The figure shows three views and two pictorial views of one solid part (mm, origin at its lowest corner). Answer the questions. Coordinates: 2 decimals unless noted, no trailing zeros. Write each loop counter-clockwise with the first axis right and the second up, starting at its lowest first coordinate (ties: lowest second). Pieces come first, ordered by that corner, then holes.
Item 1: Determine the mould class of the marked faces 1 and 2 for opening direction Z: released by +Z, released by -Z, zero draft, split by the parting line, or undercut.
Item 2: Section C-C (y = 1.65) is taken. Give the vertices of the cut face in (x, z), then the cut area to 3 significant figures.
Item 3: Section B-B (x = 20) is taken. Give the vertices of the cut face in (y, z), then the cut area to 3 significant figures.
Item 4: Straight lines are drawn through the part: probe 1 along X at (y, z) = (1.35, 5); probe 2 along X at (y, z) = (1.55, 19.5); probe 3 along X at (y, z) = (0.7, 35). For each, find the intervals that lie inside material, in ascending order.
Item 5: Section A-A (z = 20) is taken. Give the vertices of the cut face in (x, y), then the cut area to 3 significant figures.
Item 6: Each of these flat-tipped pins is pushed along its axis until it touches: P1, Ø2, axis at x = 35, z = 35, coming from the -Y side; P2, Ø1, axis at x = 31, z = 8.5, coming from the +Y side. Where does it stop, or does it pass through?
Item 7: Section D-D (x = 35) is taken. Give the vertices of the cut face in (y, z), then the cut area to 3 significant figures.
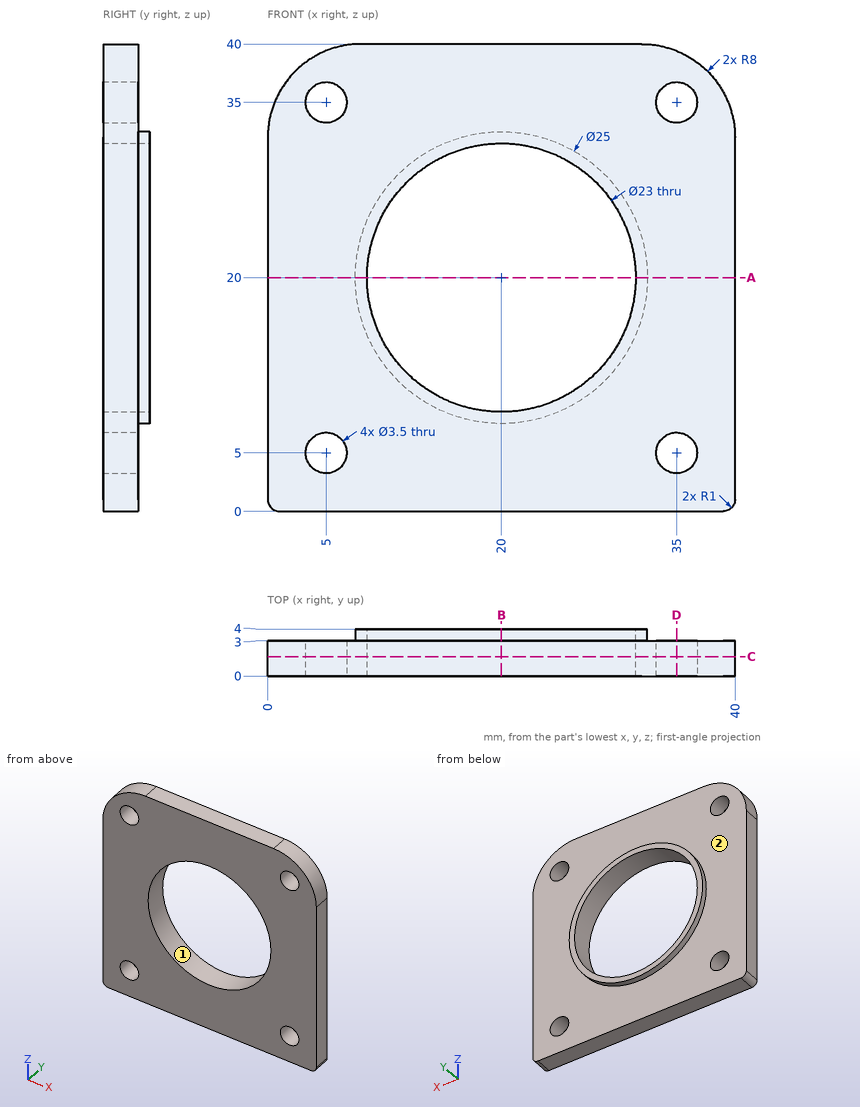
Established:
1. face 1: undercut
1. face 2: zero draft
2. outline: (0, 1) arc R1 ccw to (1, 0) - (39, 0) arc R1 ccw to (40, 1) - (40, 32) arc R8 ccw to (32, 40) - (8, 40) arc R8 ccw to (0, 32) - close; hole circle Ø3.5 at (5, 5); hole circle Ø3.5 at (5, 35); hole circle Ø23 at (20, 20); hole circle Ø3.5 at (35, 5); hole circle Ø3.5 at (35, 35)
2. area: 1,120 mm2
3. outline: (0, 0) - (3, 0) - (3, 7.5) - (4, 7.5) - (4, 8.5) - (0, 8.5) - close; (0, 31.5) - (4, 31.5) - (4, 32.5) - (3, 32.5) - (3, 40) - (0, 40) - close
3. area: 53.0 mm2
4. probe 1: x = 0 to 3.25, 6.75 to 33.25, 36.75 to 40
4. probe 2: x = 0 to 8.51, 31.49 to 40
4. probe 3: x = 0.58 to 3.25, 6.75 to 33.25, 36.75 to 39.42
5. outline: (0, 0) - (8.5, 0) - (8.5, 4) - (7.5, 4) - (7.5, 3) - (0, 3) - close; (31.5, 0) - (40, 0) - (40, 3) - (32.5, 3) - (32.5, 4) - (31.5, 4) - close
5. area: 53.0 mm2
6. P1: passes through
6. P2: stops at y = 3
7. outline: (0, 0) - (3, 0) - (3, 3.25) - (0, 3.25) - close; (0, 6.75) - (3, 6.75) - (3, 33.25) - (0, 33.25) - close; (0, 36.75) - (3, 36.75) - (3, 39.42) - (0, 39.42) - close
7. area: 97.2 mm2
